from build123d import *

# Parameters (mm, degrees)
SKETCH1_W                = 460
SKETCH1_H                = 88.9
BOSS_EXTRUDE1_DEPTH      = 38.1
SKETCH2_W                = 38.1
SKETCH2_H                = 88.9
BOSS_EXTRUDE2_DEPTH      = 910
SKETCH3_W                = 38.1
SKETCH3_H                = 88.9
BOSS_EXTRUDE3_DEPTH      = 577.85
SKETCH4_W                = 38.1
SKETCH4_H                = 91.631294093
BOSS_EXTRUDE4_DEPTH      = 615
BOSS_EXTRUDE4_DEPTH_BACK = 88.9
SKETCH5_W                = 91.631294093
SKETCH5_H                = 38.1
BOSS_EXTRUDE5_DEPTH      = 460
SKETCH7_W                = 460
SKETCH7_H                = 424.5
SKETCH7_W_2              = 38.1
SKETCH7_H_2              = 152.4
CUT_EXTRUDE1_DEPTH       = 577.85
SKETCH8_W                = 88.9
SKETCH8_H                = 38.1
BOSS_EXTRUDE6_DEPTH      = 383.8
SKETCH10_R               = 10
CUT_EXTRUDE2_DEPTH       = 38.1
SKETCH9_R                = 10
CUT_EXTRUDE3_DEPTH       = 38.1


with BuildPart() as part:
    # Sketch1 → Boss-Extrude1 (new body)
    with BuildSketch(Plane(origin=(0, 0, 0), x_dir=(1, 0, 0), z_dir=(0, 1, 0))):
        Rectangle(SKETCH1_W, SKETCH1_H)
    extrude(amount=BOSS_EXTRUDE1_DEPTH)

    # Sketch2 → Boss-Extrude2 (add)
    with BuildSketch(Plane(origin=(0, 38.1, 0), x_dir=(1, 0, 0), z_dir=(0, 1, 0))):
        with Locations((-210.95, 0)):
            Rectangle(SKETCH2_W, SKETCH2_H)
        with Locations((210.95, 0)):
            Rectangle(SKETCH2_W, SKETCH2_H)
    extrude(amount=BOSS_EXTRUDE2_DEPTH)

    # Sketch3 → Boss-Extrude3 (add)
    with BuildSketch(Plane(origin=(0, 0, -44.45), x_dir=(-1, 0, 0), z_dir=(0, 0, -1))):
        with Locations((210.95, 992.55)):
            Rectangle(SKETCH3_W, SKETCH3_H)
        with Locations((-210.95, 992.55)):
            Rectangle(SKETCH3_W, SKETCH3_H)
    extrude(amount=-BOSS_EXTRUDE3_DEPTH)

    # Sketch4 → Boss-Extrude4 (add, two sides)
    with BuildSketch(Plane.XZ.offset(-948.1)) as boss_extrude4_sk:
        with Locations((-249.05, 487.584352954)):
            Rectangle(SKETCH4_W, SKETCH4_H)
        with Locations((249.05, 487.584352954)):
            Rectangle(SKETCH4_W, SKETCH4_H)
    extrude(amount=BOSS_EXTRUDE4_DEPTH)
    extrude(boss_extrude4_sk.sketch, amount=-BOSS_EXTRUDE4_DEPTH_BACK)

    # Sketch5 → Boss-Extrude5 (add)
    with BuildSketch(Plane.ZY.offset(-230)):
        with Locations((487.584352954, 352.15)):
            Rectangle(SKETCH5_W, SKETCH5_H)
    extrude(amount=BOSS_EXTRUDE5_DEPTH)

    # Sketch7 → Cut-Extrude1 (cut)
    with BuildSketch(Plane.XY.offset(533.4)):
        with Locations((0, 583.45)):
            Rectangle(SKETCH7_W, SKETCH7_H)
        Polygon((268.1, -246.273106328), (268.1, 333.1), (-268.1, 333.1), (-268.1, 795.7), (-577.367310112, 795.7), (-577.367310112, -246.273106328), align=None)
        Polygon((268.1, 333.1), (268.1, 795.7), (230, 795.7), (230, 371.2), (-230, 371.2), (-230, 795.7), (-268.1, 795.7), (-268.1, 333.1), align=None)
        with Locations((249.05, 871.9)):
            Rectangle(SKETCH7_W_2, SKETCH7_H_2)
        with Locations((-249.05, 871.9)):
            Rectangle(SKETCH7_W_2, SKETCH7_H_2)
    extrude(amount=-CUT_EXTRUDE1_DEPTH, mode=Mode.SUBTRACT)

    # Sketch8 → Boss-Extrude6 (add)
    with BuildSketch(Plane(origin=(-191.9, 0, 0), x_dir=(0, 0, -1), z_dir=(1, 0, 0))):
        with Locations((0, 814.75)):
            Rectangle(SKETCH8_W, SKETCH8_H)
        with Locations((-488.95, 967.15)):
            Rectangle(SKETCH8_W, SKETCH8_H)
    extrude(amount=BOSS_EXTRUDE6_DEPTH)

    # Sketch10 → Cut-Extrude2 (cut)
    with BuildSketch(Plane.XZ.offset(-948.1)):
        with Locations((-141.1, 488.95)):
            Circle(SKETCH10_R)
        with Locations((141.1, 488.95)):
            Circle(SKETCH10_R)
    extrude(amount=-CUT_EXTRUDE2_DEPTH, mode=Mode.SUBTRACT)

    # Sketch9 → Cut-Extrude3 (cut)
    with BuildSketch(Plane.XZ.offset(-795.7)):
        Circle(SKETCH9_R)
    extrude(amount=-CUT_EXTRUDE3_DEPTH, mode=Mode.SUBTRACT)


solid = part.part
The listing builds one solid part. Answer for the finished solid, in the listing's coordinates (mm). A direction names the side the tool comes from. Give positions to 0.01 mm unless a question says otherwise; leave off trailing zeros. Write each loop counter-clockwise with the first axis right and the second up, starting at its lowest first coordinate (ties: lowest second). Pieces come first, ordered by that corner, then holes.
Item 1: Find the intervals of material crossed by line 1 along X through (y, z) = (967, 488); line 2 along Z through (x, y) = (-141, 977); line 3 along X through (y, z) = (995, 156), in increasing order.
Item 2: Determine the mould class of faces 5 (the flat face through (-214, 1037, 249)), 6 (the flat face through (230, 968, 148)), 7 (the flat face through (-3, 833.8, 11)) for opening direction X: released by +X, released by -X, zero draft, split by the parting line, or undercut.
Item 3: Section C-C, the plane z = 149 is taken. Write down the section's boundary in (x, y), plus the area to 3 significant figures.
Item 4: Section B-B, the plane x = 141.1 is taken. Write down the section's boundary in (y, z), plus the area to 3 significant figures.
Item 5: Flat-ended cylindrical pins translate along their axes: P1, Ø12, axis at x = 196, z = 304.5, coming from the -Y side; P2, Ø16, axis at x = -141.1, z = 488.95, coming from the -Y side; P3, Ø11.5, axis at x = -50, y = 961, coming from the -Z side; P4, Ø19, axis at x = -245, y = 978, coming from the -Z side. Find the tip coordinate at first contact, or state that the pin passes through.
Item 6: Section D-D, the plane z = 488.95 is taken. Write down the section's boundary in (x, y).
Item 7: Section A-A, the plane y = 919 is taken. Write down the section's boundary in (x, z).
Item 8: Which of the six approach directions +Z, -Z, +X, -X, +Y, -Y give full straight-line access (tool end or side, diameter ignored) to faces 1 (the flat face through (-3, 967, 444.5)), 2 (the flat face through (-3, 986.2, 490)), 3 (the flat face through (-191.9, 979, 176)), 4 (the flat face through (-249, 992, 441.769))?
Completed:
1. line 1: x = -268.1 to -151.05, -131.15 to 131.15, 151.05 to 268.1
1. line 2: z = 444.5 to 478.95, 498.95 to 533.4
1. line 3: x = -230 to -191.9, 191.9 to 230
2. face 5: zero draft
2. face 6: released by +X
2. face 7: undercut
3. outline: (-230, 948.1) - (-191.9, 948.1) - (-191.9, 1037) - (-230, 1037) - close; (191.9, 948.1) - (230, 948.1) - (230, 1037) - (191.9, 1037) - close
3. area: 6,770 mm2
4. outline: (795.7, -44.45) - (833.8, -44.45) - (833.8, 44.45) - (795.7, 44.45) - close; (948.1, 444.5) - (986.2, 444.5) - (986.2, 478.95) - (948.1, 478.95) - close; (948.1, 498.95) - (986.2, 498.95) - (986.2, 533.4) - (948.1, 533.4) - close
4. area: 6,010 mm2
5. P1: stops at y = 948.1
5. P2: passes through
5. P3: stops at z = 444.5
5. P4: stops at z = 441.77
6. outline: (-268.1, 948.1) - (-151.1, 948.1) - (-151.1, 986.2) - (-191.9, 986.2) - (-191.9, 1037) - (-268.1, 1037) - close; (-131.1, 948.1) - (131.1, 948.1) - (131.1, 986.2) - (-131.1, 986.2) - close; (151.1, 948.1) - (268.1, 948.1) - (268.1, 1037) - (191.9, 1037) - (191.9, 986.2) - (151.1, 986.2) - close
7. outline: (-230, -44.45) - (-191.9, -44.45) - (-191.9, 44.45) - (-230, 44.45) - close; (191.9, -44.45) - (230, -44.45) - (230, 44.45) - (191.9, 44.45) - close
8. face 1: -Z, +Y, -Y
8. face 2: +Z, -Z, +Y
8. face 3: -Z, +Y
8. face 4: -Z, -X, +Y, -Y
